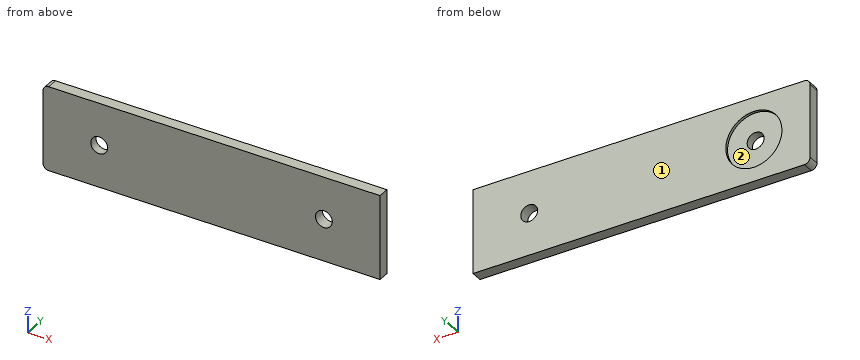
from build123d import *

# Parameters (mm, degrees)
BOSS_EXTRUDE1_DEPTH = 2
SKETCH2_R           = 5
CUT_EXTRUDE1_DEPTH  = 0.5
FILLET1_R           = 1


with BuildPart() as part:
    # Sketch1 → Boss-Extrude1 (new body)
    with BuildSketch(Plane(origin=(0, 0, 0), x_dir=(1, 0, 0), z_dir=(0, 1, 0))):
        with BuildLine():
            Line((60, 7.5), (51.5, 7.5))
            ThreePointArc((51.5, 7.5), (50, 6), (48.5, 7.5))
            Line((48.5, 7.5), (11.5, 7.5))
            ThreePointArc((11.5, 7.5), (10, 6), (8.5, 7.5))
            Line((8.5, 7.5), (0, 7.5))
            Line((0, 7.5), (0, 0))
            Line((0, 0), (60, 0))
            Line((60, 0), (60, 7.5))
        make_face()
        with BuildLine():
            ThreePointArc((48.5, 7.5), (50, 9), (51.5, 7.5))
            Line((51.5, 7.5), (60, 7.5))
            Line((60, 7.5), (60, 15))
            Line((60, 15), (0, 15))
            Line((0, 15), (0, 7.5))
            Line((0, 7.5), (8.5, 7.5))
            ThreePointArc((8.5, 7.5), (10, 9), (11.5, 7.5))
            Line((11.5, 7.5), (48.5, 7.5))
        make_face()
    extrude(amount=BOSS_EXTRUDE1_DEPTH)

    # Sketch2 → Cut-Extrude1 (cut)
    with BuildSketch(Plane(origin=(0, 2, 0), x_dir=(1, 0, 0), z_dir=(0, 1, 0))):
        with Locations(Location((10, 7.5, 0), (0, 0, 270))):
            Circle(SKETCH2_R)
    extrude(amount=-CUT_EXTRUDE1_DEPTH, mode=Mode.SUBTRACT)

    # Fillet1
    fillet1_edges = [part.edges().sort_by_distance(p)[0] for p in [
        (0, 1, 0),
        (0, 1, -15),
    ]]
    fillet(fillet1_edges, radius=FILLET1_R)


solid = part.part
The listing builds one solid part. Answer for the finished solid, in the listing's coordinates (mm). Face numbers are marked on the shaded views. Coordinates: 2 decimals unless noted, no trailing zeros. Order: outer loops, then holes, each group sorted by start corner. A loop starts at its lowest first (then second) coordinate and runs counter-clockwise, first axis right, second up.
Q1. A cutting plane is placed at A-A, the plane x = 10. Write down the section's boundary in (y, z), and give its area (3 significant figures).
Q2. A cutting plane is placed at B-B, the plane y = 0.35. Write down the section's boundary in (x, z).
Q3. Consider line 1 (X direction, y = 0.45, z = -7.5); line 2 (X direction, y = 1.85, z = -7.5); line 3 (Z direction, x = 50, y = 1.3). Determine where each line is inside the solid, lowest interval first.
Q4. For a pull along Z with two mould halves and no side action, classify the marked faces 1 and 2 as pulls with the +Z half, pulls with the -Z half, needs draft (parallel to the pull), parting line crosses it, or undercut.
Q5. A cutting plane is placed at C-C, the plane z = -7.5. Write down the section's boundary in (x, y).
Q6. A cutting plane is placed at D-D, the plane x = 50. Write down the section's boundary in (y, z).
Q7. Given P1, Ø3, axis at x = 8.5, z = -10, coming from the +Y side, flat-ended and moving along its own axis, determine where the tip first touches the part or whether it passes through.
Answers follow:
1. outline: (0, -15) - (2, -15) - (2, -12.5) - (1.5, -12.5) - (1.5, -9) - (0, -9) - close; (0, -6) - (1.5, -6) - (1.5, -2.5) - (2, -2.5) - (2, 0) - (0, 0) - close
1. area: 20.5 mm2
2. outline: (0, -14) arc R1 ccw to (1, -15) - (60, -15) - (60, 0) - (1, 0) arc R1 ccw to (0, -1) - close; hole circle Ø3 at (10, -7.5); hole circle Ø3 at (50, -7.5)
3. line 1: x = 0 to 8.5, 11.5 to 48.5, 51.5 to 60
3. line 2: x = 0 to 5, 15 to 48.5, 51.5 to 60
3. line 3: z = -15 to -9, -6 to 0
4. face 1: needs draft
4. face 2: undercut
5. outline: (0, 0) - (8.5, 0) - (8.5, 1.5) - (5, 1.5) - (5, 2) - (0, 2) - close; (11.5, 0) - (48.5, 0) - (48.5, 2) - (15, 2) - (15, 1.5) - (11.5, 1.5) - close; (51.5, 0) - (60, 0) - (60, 2) - (51.5, 2) - close
6. outline: (0, -15) - (2, -15) - (2, -9) - (0, -9) - close; (0, -6) - (2, -6) - (2, 0) - (0, 0) - close
7. P1: stops at y = 1.5
